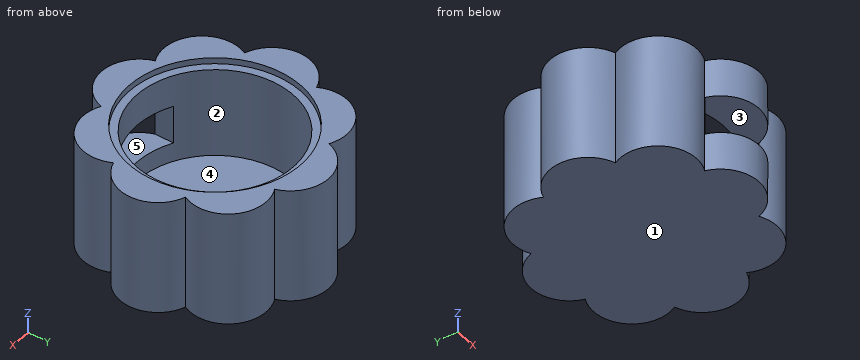
Autodesk Fusion 360 part; units mm, degrees
sketch "Boceto1" plane through (0, 0, 0) normal (0, 0, 1) x (1, 0, 0)
  circle A0 centre (0, 0) radius 41
  circle A1 centre (0, 0) radius 50
  circle A2 centre (0, 0) radius 45
  arc A3 (-19.068, 46.0342) -> (-46.0342, 19.068) centre (-28.2843, 28.2843) ccw
  arc A4 (-46.0342, -19.068) -> (-19.068, -46.0342) centre (-28.2843, -28.2843) ccw
  arc A5 (-46.0342, 19.068) -> (-46.0342, -19.068) centre (-40, 0) ccw
  arc A6 (-19.068, -46.0342) -> (19.068, -46.0342) centre (0, -40) ccw
  arc A7 (46.0342, -19.068) -> (46.0342, 19.068) centre (40, 0) ccw
  arc A8 (19.068, -46.0342) -> (46.0342, -19.068) centre (28.2843, -28.2843) ccw
  arc A9 (19.068, 46.0342) -> (-19.068, 46.0342) centre (0, 40) ccw
  arc A10 (46.0342, 19.068) -> (19.068, 46.0342) centre (28.2843, 28.2843) ccw
  dimension "d1" = 82
  dimension "d2" = 100
  dimension "d3" = 90
extrude "Extruir1" add sketch "Boceto1" along normal blind 10 contours A0
extrude "Extruir2" add sketch "Boceto1" along normal blind 56.8 contours A2
extrude "Extruir3" add sketch "Boceto1" along normal blind 60 contours A1 A3 A4 A5 A6 A7 A8 A9 A10 | A1 A7 | A1 A10 | A1 A8 | A1 A9 | A1 A6 | A1 A3 | A1 A4 | A1 A5
sketch "Boceto2" plane through (0, 0, 0) normal (0, 1, 0) x (1, 0, 0)
  line L0 (-19, -20) -> (19.0938, -20)
  line L1 (19.0938, -20) -> (19.0938, -40)
  line L2 (19.0938, -40) -> (-19, -40)
  line L3 (-19, -40) -> (-19, -20)
  dimension "d15" = 20
extrude "Extruir4" cut sketch "Boceto2" against normal blind 60
Geometry check sheet. Reference: the model listing, model coordinates, mm. Face numbers are marked on the shaded views. A direction names the side the tool comes from. Round coordinates to 2 decimals unless told otherwise and drop trailing zeros. Loops run counter-clockwise (first coordinate to the right, second up) from the corner with the lowest first, then second, coordinate; pieces in that order, holes last. Notation, with made-up numbers: (31, 37.25) - (49, 37.25) arc R13 ccw to (49, 47.25) - close; hole circle Ø7 at (-34, -11). An arc over 180 degrees is marked (long way). One line per question, with ' | ' between items. Start each with the question number.
1. Cross-section at B-B on y = 0. Record the cut outline in (x, z), then the cut area to 3 significant figures.
2. Cross-section at D-D on z = 27.5. Record the cut outline in (x, y).
3. Scan lines: line 1 (Y direction, x = 0, z = 58); line 2 (Y direction, x = -7.5, z = 57.5); line 3 (Y direction, x = 0, z = 28). Record each from-to range of solid material in increasing order. Write a range as [from, to].
4. Depth check by flat-ended pin: pin 1 (2 mm diameter, centred on x = 4.5, y = 28, fed in from -Z); pin 2 (1 mm diameter, centred on y = 35.5, z = 52, fed in from -X); pin 3 (12 mm diameter, centred on x = -21.5, y = -1, fed in from +Z); pin 4 (11 mm diameter, centred on y = -43, z = 32, fed in from +X). Enter the tip coordinate at first touch or a pass-through.
5. Cross-section at A-A on z = 53. Record the cut outline in (x, y).
6. Cross-section at C-C on x = -21. Record the cut outline in (y, z), then the cut area to 3 significant figures.
7. Draft check along Y on the marked faces 4 and 5. Enter one of: released by +Y, released by -Y, zero draft, split by the parting line, or undercut.
8. Tool access check on the marked faces 1, 2 and 3. Record the directions out of +Z, -Z, +X, -X, +Y, -Y that give a thin tool (end or side, any length) a straight path to the whole face; none if there is none.
Taken from the geometry:
1) outline: (-60, 0) - (60, 0) - (60, 60) - (45, 60) - (45, 56.8) - (41, 56.8) - (41, 10) - (-41, 10) - (-41, 56.8) - (-45, 56.8) - (-45, 60) - (-60, 60) - close | area: 3,070 mm²
2) outline: (-46.03, -19.07) arc R20 ccw to (-19.07, -46.03) arc R20 ccw to (-19, -46.25) - (-19, -36.33) arc R41 cw (long way) to (19.09, -36.28) - (19.09, -46.05) arc R20 ccw to (46.03, -19.07) arc R20 ccw to (46.03, 19.07) arc R20 ccw to (19.07, 46.03) arc R20 ccw to (-19.07, 46.03) arc R20 ccw to (-46.03, 19.07) arc R20 ccw to start
3) line 1: [-60, -45], [45, 60] | line 2: [-58.54, -44.37], [44.37, 58.54] | line 3: [41, 60]
4) pin 1: z = 0 | pin 2: x = -47.12 | pin 3: z = 10 | pin 4: x = 46.03
5) outline: (-46.03, -19.07) arc R20 ccw to (-19.07, -46.03) arc R20 ccw to (19.07, -46.03) arc R20 ccw to (46.03, -19.07) arc R20 ccw to (46.03, 19.07) arc R20 ccw to (19.07, 46.03) arc R20 ccw to (-19.07, 46.03) arc R20 ccw to (-46.03, 19.07) arc R20 ccw to start; hole circle Ø82 at (0, 0)
6) outline: (-46.91, 0) - (46.91, 0) - (46.91, 60) - (39.8, 60) - (39.8, 56.8) - (35.21, 56.8) - (35.21, 10) - (-35.21, 10) - (-35.21, 56.8) - (-39.8, 56.8) - (-39.8, 60) - (-46.91, 60) - close | area: 2,080 mm²
7) face 4: undercut | face 5: zero draft
8) face 1: -Z, +X, -X, +Y, -Y | face 2: +Z | face 3: -Y
